Verification items for the finished model (mm, model axes). Give positions to 0.01 mm unless a question says otherwise; leave off trailing zeros. Write each loop counter-clockwise with the first axis right and the second up, starting at its lowest first coordinate (ties: lowest second). Pieces come first, ordered by that corner, then holes. Notation, with made-up numbers: M 43.5,73 L 54.5,73 A13 ccw 54.5,95 Z; hole C 4.5,88.5 d4. An arc over 180 degrees is marked long. Write item = value, one per line.
from build123d import *

# Parameters (mm, degrees)
BOSS_EXTRUDE1_DEPTH = 4.5
FILLET1_R           = 5


with BuildPart() as part:
    # Sketch1 → Boss-Extrude1 (new body)
    with BuildSketch(Plane.XY):
        Polygon((0, 137.753787975), (74.246212025, 212), (225.753787975, 212), (300, 137.753787975), (300, 0), (0, 0), align=None)
    extrude(amount=BOSS_EXTRUDE1_DEPTH)

    # Fillet1
    fillet1_edges = [part.edges().sort_by_distance(p)[0] for p in [
        (74.246212025, 212, 2.25),
        (225.753787975, 212, 2.25),
        (300, 137.753787975, 2.25),
        (300, 0, 2.25),
        (0, 0, 2.25),
    ]]
    fillet(fillet1_edges, radius=FILLET1_R)


solid = part.part
1) Material ranges on probe 1 along Y at (x, z) = (26, 2.1); probe 2 along X at (y, z) = (200, 4.1); probe 3 along Y at (x, z) = (235, 2.8), recorded low to high. Write a range as from..to.
From the geometry:
probe_1 = 0..163.75
probe_2 = 62.25..237.75
probe_3 = 0..202.75
2) Cross-section at A-A on z = 1.7. Record the boundary of the cut face in (x, y), plus the area to 3 significant figures.
From the geometry:
outline = M 0,5 A5 ccw 5,0 L 295,0 A5 ccw 300,5 L 300,135.68 A5 ccw 298.54,139.22 L 227.22,210.54 A5 ccw 223.68,212 L 76.32,212 A5 ccw 72.78,210.54 L 0,137.75 Z
area = 58,100 mm^2
3) Cross-section at B-B on y = 166.5. Record the boundary of the cut face in (x, z), plus the area to 3 significant figures.
From the geometry:
outline = M 28.75,0 L 271.25,0 L 271.25,4.5 L 28.75,4.5 Z
area = 1,090 mm^2
4) Cross-section at C-C on x = 58.5. Record the boundary of the cut face in (y, z).
From the geometry:
outline = M 0,0 L 196.25,0 L 196.25,4.5 L 0,4.5 Z
